from build123d import *

# Parameters (mm, degrees)
BOSS_EXTRU_1_DEPTH      = 11.9
BOSS_EXTRU_2_DEPTH      = 10.1
BOSS_EXTRU_3_DEPTH      = 10.6
ESQUISSE4_R             = 16.25
ENL_V_MAT_EXTRU_1_DEPTH = 0.5
ESQUISSE5_R             = 11
BOSS_EXTRU_4_DEPTH      = 1.7
ESQUISSE6_R             = 2.5
BOSS_EXTRU_5_DEPTH      = 22.2
CHANFREIN1_SIZE         = 0.3
ENL_V_MAT_EXTRU_2_DEPTH = 16
ESQUISSE8_R             = 1
ENL_V_MAT_EXTRU_3_DEPTH = 7


with BuildPart() as part:
    # Esquisse1 → Boss.-Extru.1 (new body)
    with BuildSketch(Plane.XY):
        Polygon((21, -16.9), (21, 16.9), (16.9, 21), (-16.9, 21), (-21, 16.9), (-21, -16.9), (-16.9, -21), (16.9, -21), align=None)
    extrude(amount=BOSS_EXTRU_1_DEPTH)

    # Esquisse2 → Boss.-Extru.2 (add)
    with BuildSketch(Plane.XY.offset(11.9)):
        Polygon((14, 21), (21, 14), (21, -14), (14, -21), (-14, -21), (-21, -14), (-21, 14), (-14, 21), align=None)
    extrude(amount=BOSS_EXTRU_2_DEPTH)

    # Esquisse3 → Boss.-Extru.3 (add)
    with BuildSketch(Plane.XY.offset(22)):
        Polygon((16.9, 21), (21, 16.9), (21, -16.9), (16.9, -21), (-16.9, -21), (-21, -16.9), (-21, 16.9), (-16.9, 21), align=None)
    extrude(amount=BOSS_EXTRU_3_DEPTH)

    # Esquisse4 → Enlèv. mat.-Extru.1 (cut)
    with BuildSketch(Plane.XY.offset(32.6)):
        Circle(ESQUISSE4_R)
    extrude(amount=-ENL_V_MAT_EXTRU_1_DEPTH, mode=Mode.SUBTRACT)

    # Esquisse5 → Boss.-Extru.4 (add)
    with BuildSketch(Plane.XY.offset(32.1)):
        Circle(ESQUISSE5_R)
    extrude(amount=BOSS_EXTRU_4_DEPTH)

    # Esquisse6 → Boss.-Extru.5 (add)
    with BuildSketch(Plane.XY.offset(33.8)):
        Circle(ESQUISSE6_R)
    extrude(amount=BOSS_EXTRU_5_DEPTH)

    # Chanfrein1
    chanfrein1_edges = [part.edges().sort_by_distance(p)[0] for p in [
        (-2.5, 0, 56),
    ]]
    chamfer(chanfrein1_edges, length=CHANFREIN1_SIZE)

    # Esquisse7 → Enlèv. mat.-Extru.2 (cut)
    with BuildSketch(Plane.XY.offset(56)):
        with BuildLine():
            Line((2, 1.5), (2, -1.5))
            ThreePointArc((2, -1.5), (2.5, 0), (2, 1.5))
        make_face()
    extrude(amount=-ENL_V_MAT_EXTRU_2_DEPTH, mode=Mode.SUBTRACT)

    # Esquisse8 → Enlèv. mat.-Extru.3 (cut)
    with BuildSketch(Plane.XY.offset(32.6)):
        with Locations((-16.8, 16.8)):
            Circle(ESQUISSE8_R)
        with Locations((-16.8, -16.8)):
            Circle(ESQUISSE8_R)
        with Locations((16.8, -16.8)):
            Circle(ESQUISSE8_R)
        with Locations((16.8, 16.8)):
            Circle(ESQUISSE8_R)
    extrude(amount=-ENL_V_MAT_EXTRU_3_DEPTH, mode=Mode.SUBTRACT)


solid = part.part
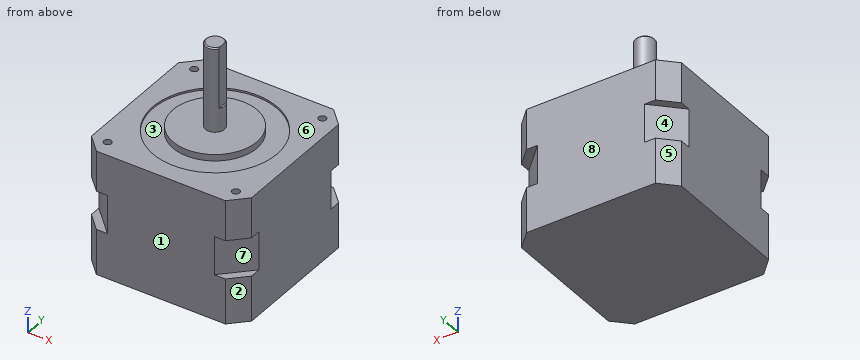
Could you check a few things on this model? Use its own coordinates, in mm. Face numbers are marked on the shaded views. A direction names the side the tool comes from. Round coordinates to 2 decimals unless told otherwise and drop trailing zeros. Order: outer loops, then holes, each group sorted by start corner. A loop starts at its lowest first (then second) coordinate and runs counter-clockwise, first axis right, second up. Notation, with made-up numbers: M -7.5,-7 L 1.5,-7 A27 ccw 1.5,13 Z; hole C 43.25,16.5 d1. An arc over 180 degrees is marked long. One line per item, written item: value.
(1) Imagine slicing it at D-D (y = 4). Write out the boundary of the cut face in (x, z), and give its area (3 significant figures).
Ans:
outline: M -21,0 L 21,0 L 21,32.6 L 15.75,32.6 L 15.75,32.1 L 10.25,32.1 L 10.25,33.8 L -10.25,33.8 L -10.25,32.1 L -15.75,32.1 L -15.75,32.6 L -21,32.6 Z
area: 1,390 mm^2
(2) I need wall thicknesses on line 1 along Y through (x, z) = (16.8, 29.5); line 2 along Z through (x, y) = (7.5, 12.5); line 3 along Z through (x, y) = (-2.5, 2.5). Which ranges of each line are inside material? Lowest first, please. Write a range as from..to.
Ans:
line 1: y = -21..-17.8, -15.8..15.8, 17.8..21
line 2: z = 0..32.1
line 3: z = 0..33.8
(3) If we mould it in two halves opening along X, with no side actions, what happens to the marked faces 1, 2 and 3? For each: released by +X, released by -X, zero draft, split by the parting line, or undercut.
Ans:
face 1: zero draft
face 2: released by +X
face 3: undercut
(4) Imagine slicing it at A-A (z = 29.5). Write out the boundary of the cut face in (x, y), and give its area (3 significant figures).
Ans:
outline: M -21,-16.9 L -16.9,-21 L 16.9,-21 L 21,-16.9 L 21,16.9 L 16.9,21 L -16.9,21 L -21,16.9 Z; hole C -16.8,-16.8 d2; hole C -16.8,16.8 d2; hole C 16.8,-16.8 d2; hole C 16.8,16.8 d2
area: 1,720 mm^2
(5) Which directions (+Z, -Z, +X, -X, +Y, -Y) give clear straight access to the entire face, cutting with the end or side of a thin tool? Please do the marked faces 4, 5, 6, 7 and 8.
Ans:
face 4: -X, +Y
face 5: +Z, -Z, -X, +Y
face 6: +Z
face 7: +X, -Y
face 8: +Z, -Z, +X, -X, +Y
(6) Imagine slicing it at C-C (z = 5). Write out the boundary of the cut face in (x, y).
Ans:
outline: M -21,-16.9 L -16.9,-21 L 16.9,-21 L 21,-16.9 L 21,16.9 L 16.9,21 L -16.9,21 L -21,16.9 Z
(7) I'm going to push flat-ended pins straight in: P1, Ø0.6, axis at x = -17, y = 16.5, coming from the +Z side; P2, Ø3, axis at x = -7.5, y = 2.5, coming from the +Z side; P3, Ø7.5, axis at x = -18, y = -19, coming from the +Z side. Where does each tip first touch, or does it pass through?
Ans:
P1: stops at z = 25.6
P2: stops at z = 33.8
P3: stops at z = 32.6
(8) Imagine slicing it at B-B (x = -13). Write out the boundary of the cut face in (y, z), and give its area (3 significant figures).
Ans:
outline: M -21,0 L 21,0 L 21,32.6 L 9.75,32.6 L 9.75,32.1 L -9.75,32.1 L -9.75,32.6 L -21,32.6 Z
area: 1,360 mm^2
